```python
from build123d import *

# Parameters (mm, degrees)
SKETCH1_W           = 22
SKETCH1_H           = 22
BOSS_EXTRUDE1_DEPTH = 3
SKETCH2_R           = 2
BOSS_EXTRUDE2_DEPTH = 14.5
SKETCH3_R           = 2
BOSS_EXTRUDE3_DEPTH = 2.75
BOSS_EXTRUDE3_TAPER = 10
BOSS_EXTRUDE4_DEPTH = 14.5
BOSS_EXTRUDE5_DEPTH = 14.5
SKETCH6_W           = 22
SKETCH6_H           = 22
BOSS_EXTRUDE6_DEPTH = 14.5


with BuildPart() as part:
    # Sketch1 → Boss-Extrude1 (new body)
    with BuildSketch(Plane(origin=(0, 0, 0), x_dir=(1, 0, 0), z_dir=(0, 1, 0))):
        Rectangle(SKETCH1_W, SKETCH1_H)
    extrude(amount=BOSS_EXTRUDE1_DEPTH)

    # Sketch2 → Boss-Extrude2 (add)
    with BuildSketch(Plane(origin=(0, 3, 0), x_dir=(1, 0, 0), z_dir=(0, 1, 0))):
        with Locations((-7.5, 7.5)):
            Circle(SKETCH2_R)
        with Locations((7.5, 7.5)):
            Circle(SKETCH2_R)
        with Locations((7.5, -7.5)):
            Circle(SKETCH2_R)
        with Locations((-7.5, -7.5)):
            Circle(SKETCH2_R)
    extrude(amount=BOSS_EXTRUDE2_DEPTH)

    # Sketch3 → Boss-Extrude3 (add)
    with BuildSketch(Plane(origin=(0, 17.5, 0), x_dir=(1, 0, 0), z_dir=(0, 1, 0))):
        with Locations((7.5, -7.5)):
            Circle(SKETCH3_R)
        with Locations((7.5, 7.5)):
            Circle(SKETCH3_R)
        with Locations((-7.5, 7.5)):
            Circle(SKETCH3_R)
        with Locations((-7.5, -7.5)):
            Circle(SKETCH3_R)
    extrude(amount=BOSS_EXTRUDE3_DEPTH, taper=BOSS_EXTRUDE3_TAPER)

    # Sketch4 → Boss-Extrude4 (add)
    with BuildSketch(Plane(origin=(0, 3, 0), x_dir=(1, 0, 0), z_dir=(0, 1, 0))):
        Polygon((-7.217157288, -7.782842712), (7.782842712, 7.217157288), (7.217157288, 7.782842712), (-7.782842712, -7.217157288), align=None)
    extrude(amount=BOSS_EXTRUDE4_DEPTH)

    # Sketch5 → Boss-Extrude5 (add)
    with BuildSketch(Plane(origin=(0, 3, 0), x_dir=(1, 0, 0), z_dir=(0, 1, 0))):
        Polygon((-7.217157288, 7.782842712), (7.782842712, -7.217157288), (7.217157288, -7.782842712), (-7.782842712, 7.217157288), align=None)
    extrude(amount=BOSS_EXTRUDE5_DEPTH)

    # Sketch6 → Boss-Extrude6 (add)
    with BuildSketch(Plane(origin=(0, 3, 0), x_dir=(1, 0, 0), z_dir=(0, 1, 0))):
        Rectangle(SKETCH6_W, SKETCH6_H)
    extrude(amount=BOSS_EXTRUDE6_DEPTH)


solid = part.part
```
Can you work these out from the model? Positions are in its coordinate system, mm. A direction names the side the tool comes from. Coordinates: 2 decimals unless noted, no trailing zeros. Write each loop counter-clockwise with the first axis right and the second up, starting at its lowest first coordinate (ties: lowest second). Pieces come first, ordered by that corner, then holes. Notation, with made-up numbers: (-28, 4) - (28, 4) arc R17 cw to (28, 31) - close; hole circle Ø1 at (78.25, 9.5). An arc over 180 degrees is marked (long way). Return JSON: item names as keys, results as strings.
Q1. I'm going to push a flat-ended pin straight in: pin 1 Ø6.5 at (x, z) = (-2.5, -3.5) entering from +Y. Where does the tip first touch, or does it pass through?
Computed values:
{"pin 1": "stops at y = 17.5"}
Q2. If we section it at C-C (x = 4): Please give me the cut outline in (y, z), then the cut area to 3 significant figures.
Computed values:
{"outline": "(0, -11) - (17.5, -11) - (17.5, 11) - (0, 11) - close", "area": "385 mm2"}
Q3. If we section it at B-B (z = -2.5): Please give me the cut outline in (x, y), then the cut area to 3 significant figures.
Computed values:
{"outline": "(-11, 0) - (11, 0) - (11, 17.5) - (-11, 17.5) - close", "area": "385 mm2"}
Q4. Thinking about a two-plate mould opening in Z: for faces 1 (the flat face through (0, 9, 11)), 2 (the conical face through (-5.93, 19.2, -6.85)), 3 (the flat face through (0, 0, 0)), 4 (the flat face through (0, 9, -11)), which applies, +Z half, -Z half, draft (parallel to the pull), parting line (faces both ways), or undercut?
Computed values:
{"face 1": "+Z half", "face 2": "undercut", "face 3": "draft", "face 4": "-Z half"}
Q5. Please list where these lines run through material, in increasing order: L1, parallel to Y at x = 3.75, z = -0.5; L2, parallel to X at y = 19, z = -8.25. Write a range as from..to.
Computed values:
{"L1": "y = 0..17.5", "L2": "x = -9.07..-5.93, 5.93..9.07"}
Q6. If we section it at A-A (x = -7.5): Please give me the cut outline in (y, z), then the cut area to 3 significant figures.
Computed values:
{"outline": "(0, -11) - (17.5, -11) - (17.5, -9.5) - (20.25, -9.02) - (20.25, -5.98) - (17.5, -5.5) - (17.5, 5.5) - (20.25, 5.98) - (20.25, 9.02) - (17.5, 9.5) - (17.5, 11) - (0, 11) - close", "area": "404 mm2"}
Q7. On a 3-axis mill with a long thin cutter (end or side, diameter ignored), from which of +Z, -Z, +X, -X, +Y, -Y can I reach the whole of each face in a straight line? I mean faces 5 (the flat face through (0, 17.5, 0)), 6 (the flat face through (11, 9, 0)). Say none if no direction works.
Computed values:
{"face 5": "+Y", "face 6": "+Z, -Z, +X, +Y, -Y"}
